```python
from build123d import *

# Parameters (mm, degrees)
SKETCH1_R               = 6.211279156
BOSS_EXTRUDE1_DEPTH     = 15
CUT_EXTRUDE1_DEPTH      = 24.031459486
CUT_EXTRUDE1_DEPTH_BACK = 24.031459486
BOSS_EXTRUDE3_DEPTH     = 1
SKETCH6_R               = 1.4
CUT_EXTRUDE2_DEPTH      = 10


with BuildPart() as part:
    # Sketch1 → Boss-Extrude1 (new body)
    with BuildSketch(Plane(origin=(0, 0, 0), x_dir=(1, 0, 0), z_dir=(0, 1, 0))):
        with BuildLine():
            Line((-3.5, 7.427994707), (-3.5, 15.427994707))
            Line((-3.5, 15.427994707), (3.5, 15.427994707))
            Line((3.5, 15.427994707), (3.5, 7.427994707))
            ThreePointArc((3.5, 7.427994707), (0, -8.211279156), (-3.5, 7.427994707))
        make_face()
        with Locations(Location((0, 0, 0), (0, 0, 270))):
            Circle(SKETCH1_R, mode=Mode.SUBTRACT)
    extrude(amount=BOSS_EXTRUDE1_DEPTH)

    # Sketch4 → Cut-Extrude1 (cut, two sides: drawn at the far end of the back side and taken through both)
    with BuildSketch(Plane(origin=(0, 15, 0), x_dir=(1, 0, 0), z_dir=(0, 1, 0)).offset(-CUT_EXTRUDE1_DEPTH_BACK)):
        with BuildLine():
            Line((-3.105639578, -5.379125539), (-4.105639578, -7.111176346))
            ThreePointArc((-4.105639578, -7.111176346), (0, -8.211279156), (4.105639578, -7.111176346))
            Line((4.105639578, -7.111176346), (3.105639578, -5.379125539))
            ThreePointArc((3.105639578, -5.379125539), (0, -6.211279156), (-3.105639578, -5.379125539))
        make_face()
    extrude(amount=CUT_EXTRUDE1_DEPTH + CUT_EXTRUDE1_DEPTH_BACK, mode=Mode.SUBTRACT)

    # Sketch5 → Boss-Extrude3 (add)
    with BuildSketch(Plane(origin=(0, 1, 0), x_dir=(-1, 0, 0), z_dir=(0, -1, 0))):
        with BuildLine():
            Line((3.105639578, -5.379125539), (2.749999992, -4.763139708))
            ThreePointArc((2.749999992, -4.763139708), (0, 5.499999985), (-2.749999992, -4.763139708))
            Line((-2.749999992, -4.763139708), (-3.105639578, -5.379125539))
            ThreePointArc((-3.105639578, -5.379125539), (0, 6.211279156), (3.105639578, -5.379125539))
        make_face()
    boss_extrude3 = extrude(amount=-BOSS_EXTRUDE3_DEPTH)

    # Mirror1: Boss-Extrude3 across plane
    add(boss_extrude3.mirror(Plane.ZX.offset(7.5)))

    # Sketch6 → Cut-Extrude2 (cut)
    with BuildSketch(Plane(origin=(0, 0, -15.427994707), x_dir=(-1, 0, 0), z_dir=(0, 0, -1))):
        with Locations((0, 7.5)):
            Circle(SKETCH6_R)
    extrude(amount=-CUT_EXTRUDE2_DEPTH, mode=Mode.SUBTRACT)


solid = part.part
```
The listing builds one solid part. Answer for the finished solid, in the listing's coordinates (mm). A direction names the side the tool comes from. Give positions to 0.01 mm unless a question says otherwise; leave off trailing zeros. Loops run counter-clockwise (first coordinate to the right, second up) from the corner with the lowest first, then second, coordinate; pieces in that order, holes last. Notation, with made-up numbers: (15.5, 79.25) - (35.5, 79.25) arc R31 cw to (35.5, 115.25) - close; hole circle Ø1 at (17.25, 78). An arc over 180 degrees is marked (long way). Return JSON: item names as keys, results as strings. Group by question number.
1. Given pin 1 Ø4 at (y, z) = (4, -11.5) entering from +X; pin 2 Ø2 at (x, y) = (4.5, 11) entering from +Z; pin 3 Ø3 at (x, z) = (-2.5, -3.5) entering from +Y, each flat-ended and moving along its own axis, determine where each tip first touches the part or whether it passes through.
2. Straight lines are drawn through the part: line 1 (Y direction, x = 0, z = -9.5); line 2 (X direction, y = 7.5, z = -9); line 3 (X direction, y = 0.35, z = 0). For each, find the intervals that lie inside material, in ascending order. Write a range as [from, to].
3. Find section D-D (z = -12.5). Write down the section's boundary in (x, y).
4. Find section C-C (y = 7.5). Write down the section's boundary in (x, z).
5. Find section A-A (z = 0). Write down the section's boundary in (x, y).
6. Determine the mould class of faces 5 (the cylindrical face through (-3.22, 7.42, -5.31)), 6 (the flat face through (-3.5, 7, -11)), 7 (the flat face through (0, 1, -6)) for opening direction Y: pulls with the +Y half, pulls with the -Y half, needs draft (parallel to the pull), parting line crosses it, or undercut.
7. Find section B-B (x = 0). Write down the section's boundary in (y, z), then the cut area to 3 significant figures.
8. Which of the six approach directions +Z, -Z, +X, -X, +Y, -Y give full straight-line access (tool end or side, diameter ignored) to faces 1 (the flat face through (0, 13, -6)), 2 (the flat face through (3.5, 7, -11)), 3 (the cylindrical face through (0.228, 14.493, -6.207)), 4 (the cylindrical face through (0.228, 0.493, -6.207))?
Verdict:
{
 "1": {"pin 1": "stops at x = 3.5", "pin 2": "stops at z = 7.11", "pin 3": "stops at y = 14"},
 "2": {"line 1": "y = [0, 6.1], [8.9, 15]", "line 2": "x = [-3.5, -1.4], [1.4, 3.5]", "line 3": "x = [-8.21, -6.21], [6.21, 8.21]"},
 "3": {"outline": "(-3.5, 0) - (3.5, 0) - (3.5, 15) - (-3.5, 15) - close; hole circle Ø2.8 at (0, 7.5)"},
 "4": {"outline": "(-4.11, 7.11) arc R8.21 ccw to (-3.5, -7.43) - (-3.5, -15.43) - (-1.4, -15.43) - (-1.4, -6.05) arc R6.21 cw to (-3.11, 5.38) - close; (1.4, -15.43) - (3.5, -15.43) - (3.5, -7.43) arc R8.21 ccw to (4.11, 7.11) - (3.11, 5.38) arc R6.21 cw to (1.4, -6.05) - close"},
 "5": {"outline": "(-8.21, 0) - (-6.21, 0) - (-6.21, 1) - (-5.5, 1) - (-5.5, 2) - (-6.21, 2) - (-6.21, 13) - (-5.5, 13) - (-5.5, 14) - (-6.21, 14) - (-6.21, 15) - (-8.21, 15) - close; (5.5, 1) - (6.21, 1) - (6.21, 0) - (8.21, 0) - (8.21, 15) - (6.21, 15) - (6.21, 14) - (5.5, 14) - (5.5, 13) - (6.21, 13) - (6.21, 2) - (5.5, 2) - close"},
 "6": {"face 5": "undercut", "face 6": "needs draft", "face 7": "pulls with the -Y half"},
 "7": {"outline": "(0, -15.43) - (6.1, -15.43) - (6.1, -6.21) - (2, -6.21) - (2, -5.5) - (1, -5.5) - (1, -6.21) - (0, -6.21) - close; (8.9, -15.43) - (15, -15.43) - (15, -6.21) - (14, -6.21) - (14, -5.5) - (13, -5.5) - (13, -6.21) - (8.9, -6.21) - close", "area": "114 mm^2"},
 "8": {"face 1": "none", "face 2": "-Z, +X, +Y, -Y", "face 3": "+Y", "face 4": "-Y"}
}
